from build123d import *

# Parameters (mm, degrees)
BOSS_EXTRUDE1_DEPTH     = 20
CUT_EXTRUDE1_DEPTH      = 58.271284253
CUT_EXTRUDE1_DEPTH_BACK = 58.271284253
SKETCH2_R               = 7.55
CUT_EXTRUDE2_DEPTH      = 58.271284253
CUT_EXTRUDE2_DEPTH_BACK = 58.271284253
SKETCH3_R               = 8.55
CUT_EXTRUDE3_DEPTH      = 40.395431329
CUT_EXTRUDE3_DEPTH_BACK = 40.395431329
SKETCH4_R               = 2.5
CUT_EXTRUDE4_DEPTH      = 40.39543138


with BuildPart() as part:
    # Sketch1 → Boss-Extrude1 (new body)
    with BuildSketch(Plane(origin=(0, 0, 0), x_dir=(1, 0, 0), z_dir=(0, 1, 0))):
        Polygon((-24, 16), (-16, 24), (16, 24), (24, 16), (24, -16), (16, -24), (-16, -24), (-24, -16), align=None)
    extrude(amount=BOSS_EXTRUDE1_DEPTH)

    # Sketch2 → Cut-Extrude1 (cut, two sides: drawn at the far end of the back side and taken through both)
    with BuildSketch(Plane.XY.offset(24).offset(-CUT_EXTRUDE1_DEPTH_BACK)):
        with Locations((0, 10)):
            Circle(SKETCH2_R)
    extrude(amount=CUT_EXTRUDE1_DEPTH + CUT_EXTRUDE1_DEPTH_BACK, mode=Mode.SUBTRACT)

    # Sketch3 → Cut-Extrude2 (cut, two sides: drawn at the far end of the back side and taken through both)
    with BuildSketch(Plane(origin=(24, 0, 0), x_dir=(0, 0, -1), z_dir=(1, 0, 0)).offset(-CUT_EXTRUDE2_DEPTH_BACK)):
        with Locations((0, 10)):
            Circle(SKETCH3_R)
    extrude(amount=CUT_EXTRUDE2_DEPTH + CUT_EXTRUDE2_DEPTH_BACK, mode=Mode.SUBTRACT)

    # Sketch4 → Cut-Extrude3 (cut, two sides: drawn at the far end of the back side and taken through both)
    with BuildSketch(Plane(origin=(0, 20, 0), x_dir=(1, 0, 0), z_dir=(0, 1, 0)).offset(-CUT_EXTRUDE3_DEPTH_BACK)):
        with Locations(Location((0, 0, 0), (0, 0, 270))):
            Circle(SKETCH4_R)
    extrude(amount=CUT_EXTRUDE3_DEPTH + CUT_EXTRUDE3_DEPTH_BACK, mode=Mode.SUBTRACT)

    # Sketch5 → Cut-Extrude4 (cut, through all)
    with BuildSketch(Plane(origin=(0, 20, 0), x_dir=(1, 0, 0), z_dir=(0, 1, 0))):
        Polygon((-24, 16), (-24, -16), (-16, -24), (16, -24), (24, -16), (24, 16), (16, 24), (-16, 24), align=None)
        Polygon((-23.8, 15.917157288), (-23.8, -15.917157288), (-15.917157288, -23.8), (15.917157288, -23.8), (23.8, -15.917157288), (23.8, 15.917157288), (15.917157288, 23.8), (-15.917157288, 23.8), align=None, mode=Mode.SUBTRACT)
    extrude(amount=-CUT_EXTRUDE4_DEPTH, mode=Mode.SUBTRACT)


solid = part.part
Read the model definition and answer for the solid it produces. Units are mm, in the model's axes. Coordinates: 2 decimals unless noted, no trailing zeros. Order: outer loops, then holes, each group sorted by start corner. A loop starts at its lowest first (then second) coordinate and runs counter-clockwise, first axis right, second up. Notation, with made-up numbers: M -35.5,-13 L 9.5,-13 A11 cw 9.5,3 Z; hole C 80,49.25 d10. An arc over 180 degrees is marked long. Put each result on its own line as item: value. Start each with the question number.
Item 1: Section C-C, the plane x = 0 is taken. Determine the outline of the cut face in (y, z), plus the area to 3 significant figures.
Item 2: Given pin 1 Ø3 at (y, z) = (13.5, 18.5) entering from -X; pin 2 Ø2 at (x, y) = (18, 9) entering from +Z, each flat-ended and moving along its own axis, determine where each tip first touches the part or whether it passes through.
Item 3: The mould has two halves that part along Z. Classify faces 1 (the face through (4, 17, -23.8)), 2 (the face through (0.751, 0.904, 2.385)), 3 (the face through (23.8, 19, 0)): +Z half, -Z half, draft (parallel to the pull), parting line (faces both ways), or undercut.
Item 4: Section B-B, the plane z = 9.5 is taken. Determine the outline of the cut face in (x, y), plus the area to 3 significant figures.
Item 5: Section A-A, the plane y = 10 is taken. Determine the outline of the cut face in (x, z).
Item 6: Consider probe 1 along Z at (x, y) = (0, 0.6); probe 2 along Y at (x, z) = (0, 18.25); probe 3 along Z at (x, y) = (11, 6). Determine where each line is inside the solid, lowest interval first. Write a range as [from, to].
Item 7: Section D-D, the plane z = 0 is taken. Determine the outline of the cut face in (x, y).
Computed:
1. outline: M 0,-23.8 L 2.45,-23.8 L 2.45,-4.01 A8.55 cw 1.82,-2.5 L 0,-2.5 Z; M 0,2.5 L 1.82,2.5 A8.55 cw 2.45,4.01 L 2.45,23.8 L 0,23.8 Z; M 17.55,-23.8 L 20,-23.8 L 20,-2.5 L 18.18,-2.5 A8.55 cw 17.55,-4.01 Z; M 17.55,4.01 A8.55 cw 18.18,2.5 L 20,2.5 L 20,23.8 L 17.55,23.8 Z
1. area: 207 mm2
2. pin 1: stops at x = -22.72
2. pin 2: stops at z = 22.72
3. face 1: -Z half
3. face 2: undercut
3. face 3: draft
4. outline: M -23.8,0 L 23.8,0 L 23.8,20 L -23.8,20 Z; hole C 0,10 d15.1
4. area: 773 mm2
5. outline: M -23.8,-15.92 L -15.92,-23.8 L -7.55,-23.8 L -7.55,-8.55 L -23.8,-8.55 Z; M -23.8,8.55 L -7.55,8.55 L -7.55,23.8 L -15.92,23.8 L -23.8,15.92 Z; M 7.55,-23.8 L 15.92,-23.8 L 23.8,-15.92 L 23.8,-8.55 L 7.55,-8.55 Z; M 7.55,8.55 L 23.8,8.55 L 23.8,15.92 L 15.92,23.8 L 7.55,23.8 Z
6. probe 1: z = [-23.8, -2.5], [2.5, 23.8]
6. probe 2: y = [0, 2.45], [17.55, 20]
6. probe 3: z = [-23.8, -7.56], [7.56, 23.8]
7. outline: M -23.8,0 L -2.5,0 L -2.5,1.45 L -23.8,1.45 Z; M -23.8,18.55 L -2.5,18.55 L -2.5,20 L -23.8,20 Z; M 2.5,0 L 23.8,0 L 23.8,1.45 L 2.5,1.45 Z; M 2.5,18.55 L 23.8,18.55 L 23.8,20 L 2.5,20 Z
